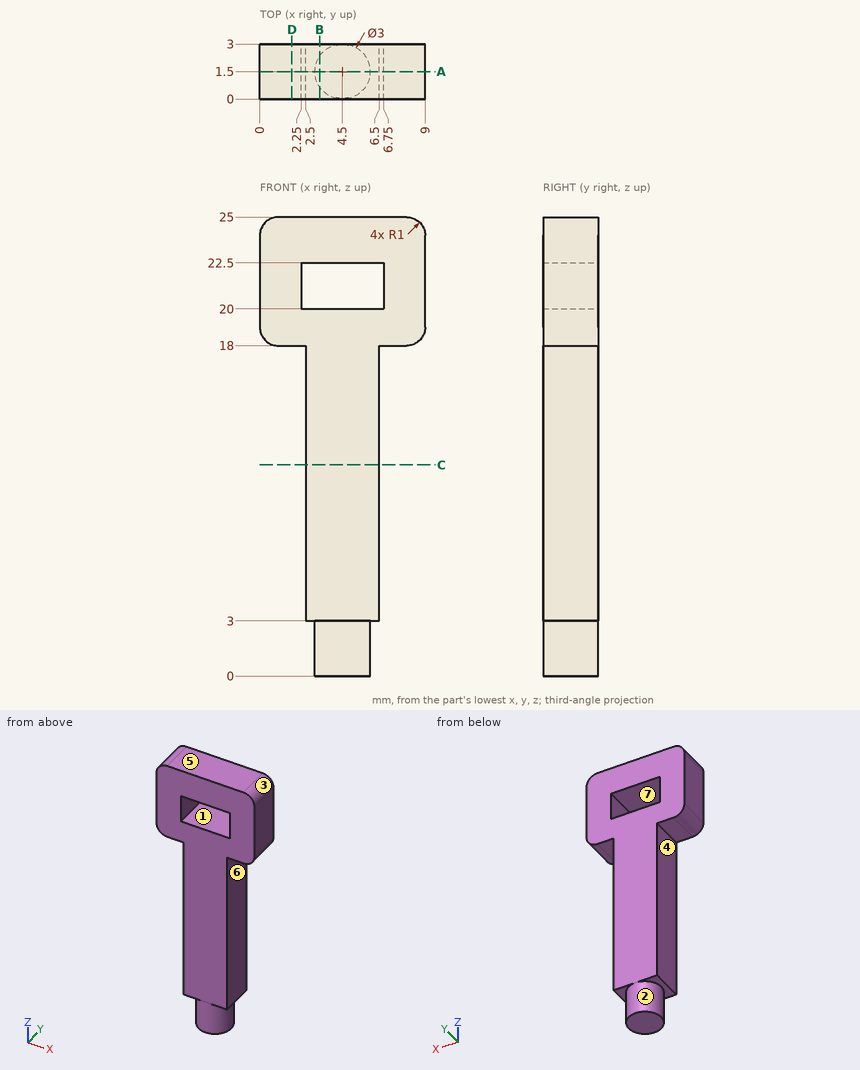
Can you work these out from the drawing? Everything is in mm from the part's minimum corner. A direction names the side the tool comes from. Round coordinates to 2 decimals unless told otherwise and drop trailing zeros. Order: outer loops, then holes, each group sorted by start corner. A loop starts at its lowest first (then second) coordinate and runs counter-clockwise, first axis right, second up. Notation, with made-up numbers: M 48.5,6.25 L 97.5,6.25 A37 cw 97.5,44.25 Z; hole C 37.5,41.5 d4. An arc over 180 degrees is marked long. Answer as CSV lines item,"result".
Item 1: Imagine slicing it at D-D on x = 1.75. List the corners of the cut face in (y, z) for me, and give its area (3 significant figures).
From the geometry:
outline,"M 0,18 L 3,18 L 3,25 L 0,25 Z"
area,"21.0 mm2"
Item 2: Which directions (+Z, -Z, +X, -X, +Y, -Y) give clear straight access to the entire face, cutting with the end or side of a thin tool? Please do the marked faces 1, 2, 3 and 4.
From the geometry:
face 1,"+Y, -Y"
face 2,"-Z"
face 3,"+Z, +X, +Y, -Y"
face 4,"-Z, -X, +Y, -Y"
Item 3: We'd pull the mould along X, two halves only. Please class the marked faces 5, 6 and 7: +X half, -X half, draft (parallel to the pull), parting line (faces both ways), or undercut.
From the geometry:
face 5,"draft"
face 6,"+X half"
face 7,"undercut"
Item 4: Please list where these lines run through material, in increasing order: L1, parallel to Z at x = 5.5, y = 2.75; L2, parallel to Z at x = 4, y = 2.25; L3, parallel to X at y = 0.9, z = 4.5. Write a range as [from, to].
From the geometry:
L1,"[3, 20], [22.5, 25]"
L2,"[0, 20], [22.5, 25]"
L3,"[2.5, 6.5]"
Item 5: Imagine slicing it at A-A on y = 1.5. List the corners of the cut face in (x, z) for me, and give its area (3 significant figures).
From the geometry:
outline,"M 0,19 A1 ccw 1,18 L 2.5,18 L 2.5,3 L 3,3 L 3,0 L 6,0 L 6,3 L 6.5,3 L 6.5,18 L 8,18 A1 ccw 9,19 L 9,24 A1 ccw 8,25 L 1,25 A1 ccw 0,24 Z; hole M 2.25,20 L 6.75,20 L 6.75,22.5 L 2.25,22.5 Z"
area,"120 mm2"
Item 6: Imagine slicing it at C-C on z = 11.5. List the corners of the cut face in (x, y) for me, and give its area (3 significant figures).
From the geometry:
outline,"M 2.5,0 L 6.5,0 L 6.5,3 L 2.5,3 Z"
area,"12.0 mm2"
Item 7: For pin 1 (1.6 mm diameter, centred on x = 2, y = 2, fed in from -Z); pin 2 (0.9 mm diameter, centred on y = 2, z = 10, fed in from +X); pin 3 (1.5 mm diameter, centred on y = 2, z = 9.5, fed in from -X), each with a flat end and sliding along its axis, tell me the tip position at first contact or that it passes through.
From the geometry:
pin 1,"z = 3"
pin 2,"x = 6.5"
pin 3,"x = 2.5"
Item 8: Imagine slicing it at B-B on x = 3.25. List the corners of the cut face in (y, z) for me.
From the geometry:
outline,"M 0,3 L 0.67,3 L 0.67,0 L 2.33,0 L 2.33,3 L 3,3 L 3,20 L 0,20 Z; M 0,22.5 L 3,22.5 L 3,25 L 0,25 Z"
